For this review, use the dimensioned drawing (mm, ordinates from the lowest corner) and the shaded views. A direction names the side the tool comes from. Coordinates: 2 decimals unless noted, no trailing zeros. Write each loop counter-clockwise with the first axis right and the second up, starting at its lowest first coordinate (ties: lowest second). Pieces come first, ordered by that corner, then holes. Notation, with made-up numbers: M -36.5,60.25 L 17.5,60.25 A12 cw 17.5,64.25 Z; hole C 73.25,45 d8. An arc over 180 degrees is marked long. Return JSON: item names as keys, results as strings.
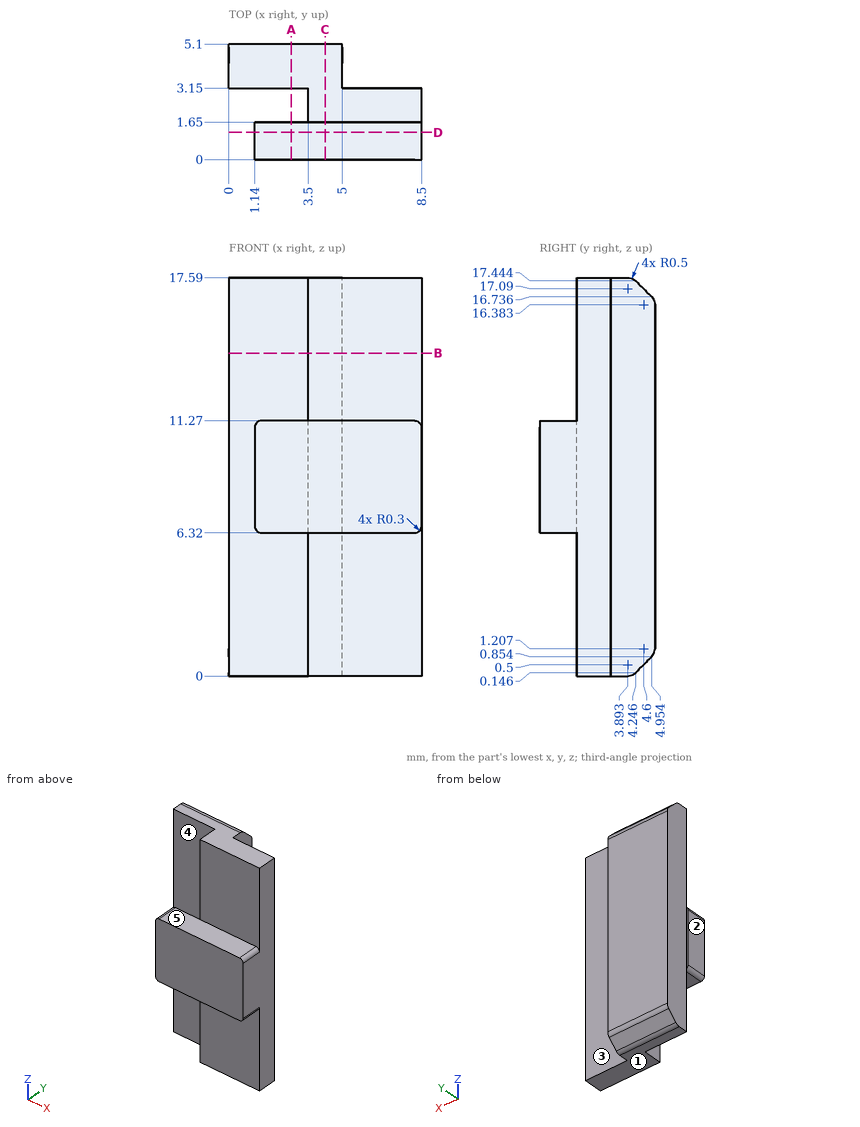
1. We need section B-B (z = 14.25). State the section outline as (x, y) points.
Checks:
{"outline": "M 0,3.15 L 3.5,3.15 L 3.5,1.65 L 8.5,1.65 L 8.5,3.15 L 5,3.15 L 5,5.1 L 0,5.1 Z"}
2. We need section C-C (x = 4.25). State the section outline as (y, z) points.
Checks:
{"outline": "M 0,6.32 L 1.65,6.32 L 1.65,0 L 3.89,0 A0.5 ccw 4.25,0.15 L 4.95,0.85 A0.5 ccw 5.1,1.21 L 5.1,16.38 A0.5 ccw 4.95,16.74 L 4.25,17.44 A0.5 ccw 3.89,17.59 L 1.65,17.59 L 1.65,11.27 L 0,11.27 Z"}
3. We need section D-D (y = 1.2). State the section outline as (x, z) points.
Checks:
{"outline": "M 1.14,6.62 A0.3 ccw 1.44,6.32 L 8.2,6.32 A0.3 ccw 8.5,6.62 L 8.5,10.97 A0.3 ccw 8.2,11.27 L 1.44,11.27 A0.3 ccw 1.14,10.97 Z"}
4. We need section A-A (x = 2.75). State the section outline as (y, z) points.
Checks:
{"outline": "M 0,6.32 L 1.65,6.32 L 1.65,11.27 L 0,11.27 Z; M 3.15,0 L 3.89,0 A0.5 ccw 4.25,0.15 L 4.95,0.85 A0.5 ccw 5.1,1.21 L 5.1,16.38 A0.5 ccw 4.95,16.74 L 4.25,17.44 A0.5 ccw 3.89,17.59 L 3.15,17.59 Z"}
5. Clearance check with flat-ended pins moving along their axes: pin 1 Ø1.6 at (y, z) = (4.5, 6) entering from +X; pin 2 Ø0.5 at (x, y) = (5.5, 1) entering from +Z; pin 3 Ø1 at (y, z) = (1, 2.5) entering from -X; pin 4 Ø1.5 at (x, z) = (7, 4.5) entering from -Y. State where each tip first meets the part, or that it passes through.
Checks:
{"pin 1": "x = 5", "pin 2": "z = 11.27", "pin 3": "through", "pin 4": "y = 1.65"}
6. Wall thickness on L1, parallel to Y at x = 3, z = 9; L2, parallel to Z at x = 5, y = 0.9; L3, parallel to Y at x = 7.75, z = 7.5: over which ranges is each line inside the solid? List them lowest first. Write a range as from..to.
Checks:
{"L1": "0..1.65, 3.15..5.1", "L2": "6.32..11.27", "L3": "0..3.15"}
7. For the marked faces 1, 2, 3, 4 and 5, list the 3-axis set-ups (+Z, -Z, +X, -X, +Y, -Y) from which the entire face can be reached by the end or side of a thin tool; tool diameter is ignored.
Checks:
{"face 1": "-Z, +X, -X, +Y, -Y", "face 2": "+Z, -Z, -X, -Y", "face 3": "+Z, -Z, +X, +Y", "face 4": "+Z, -Z, -X", "face 5": "+Z, +X, -X, -Y"}
